Work out the finished part from the listing and answer in its coordinate system (mm). Face numbers are marked on the shaded views. Coordinates: 2 decimals unless noted, no trailing zeros.
```python
from build123d import *

# Parameters (mm, degrees)
F2_W     = 4.20624
F2_H     = 20.0195648662
F2_H_2   = 4.20624
F2_W_2   = 17.6414342363
F3_DEPTH = 2.54


with BuildPart() as f1:
    # F0 (on Top) → F1 (revolve)
    with BuildSketch(Plane.XY):
        with BuildLine():
            Line((0, 36.7317478065), (0, 0))
            Line((0, 0), (14.3002, 0))
            add(Edge.make_bspline(
                [(9.5422007305, 36.7317478065), (9.8377349923, 34.8905601939), (10.3712029618, 31.5670382058), (5.4519131165, 31.1307695275), (8.3582832439, 11.1967644856), (13.374842383, 9.3400085371), (13.964740637, 3.3859269715), (14.3002, 0)],
                knots=[0, 0, 0, 0, 0.1612494868, 0.2910709431, 0.6079020726, 0.7770243936, 1, 1, 1, 1], degree=3))
            Line((9.5422007305, 36.7317478065), (0, 36.7317478065))
        make_face()
    revolve(axis=Axis((0, 18.3658739032, 0), (0, 1, 0)))

    # F2 (on face) → F3 (cut)
    with BuildSketch(Plane(origin=(0, 36.7317478065, 0), x_dir=(-1, 0, 0), z_dir=(0, 1, 0))):
        with Locations((0, -12.1129024331)):
            Rectangle(F2_W, F2_H)
        Rectangle(F2_W, F2_H_2)
        with Locations((10.9238371181, 0)):
            Rectangle(F2_W_2, F2_H_2)
        with Locations((-10.9238371181, 0)):
            Rectangle(F2_W_2, F2_H_2)
        with Locations((0, 12.1129024331)):
            Rectangle(F2_W, F2_H)
    extrude(amount=-F3_DEPTH, mode=Mode.SUBTRACT)


solid = f1.part
```
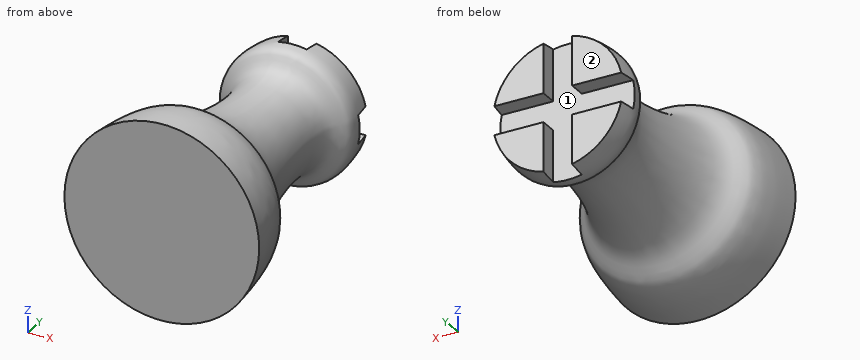
1. The mould has two halves that part along Z. Classify the marked faces 1 and 2: released by +Z, released by -Z, zero draft, split by the parting line, or undercut.
2. Consider probe 1 along Y at (x, z) = (-3.25, 1); probe 2 along X at (y, z) = (29.5, 1.25); probe 3 along Z at (x, y) = (-4.75, 32). Determine where each line is inside the solid, lowest interval first.
3. Flat-ended cylindrical pins translate along their axes: pin 1 (1.3 mm diameter, centred on y = 35, z = -4.5, fed in from -X); pin 2 (1.3 mm diameter, centred on y = 36, z = 5, fed in from -X); pin 3 (2 mm diameter, centred on x = -6, y = 36, fed in from -Z). Find the tip coordinate at first contact, or state that the pin passes through.
Worked out:
1. face 1: undercut
1. face 2: zero draft
2. probe 1: y = 0 to 34.19
2. probe 2: x = -7.14 to 7.14
2. probe 3: z = -8.13 to 8.13
3. pin 1: stops at x = -9.02
3. pin 2: stops at x = -8.64
3. pin 3: stops at z = -8.29
